```python
from build123d import *

# Parameters (mm, degrees)
SKETCH1_W           = 121
SKETCH1_H           = 25
BOSS_EXTRUDE1_DEPTH = 4
SKETCH3_W           = 10
SKETCH3_H           = 4
BOSS_EXTRUDE3_DEPTH = 4
LPATTERN2_COUNT     = 3
LPATTERN2_PITCH     = 20
LPATTERN2_COL_COUNT = 3
LPATTERN2_COL_PITCH = 20
SKETCH4_W           = 4
SKETCH4_H           = 5
BOSS_EXTRUDE4_DEPTH = 4
LPATTERN3_COUNT     = 3
LPATTERN3_PITCH     = 10


with BuildPart() as part:
    # Sketch1 → Boss-Extrude1 (new body)
    with BuildSketch(Plane(origin=(0, 0, 0), x_dir=(1, 0, 0), z_dir=(0, 1, 0))):
        with Locations((60.5, -12.5)):
            Rectangle(SKETCH1_W, SKETCH1_H)
    extrude(amount=BOSS_EXTRUDE1_DEPTH)

    # Sketch3 → Boss-Extrude3 (add, through all)
    with BuildSketch(Plane(origin=(0, 0, 0), x_dir=(-1, 0, 0), z_dir=(0, -1, 0))):
        with Locations((-60.5, 2)):
            Rectangle(SKETCH3_W, SKETCH3_H)
    boss_extrude3 = extrude(amount=-BOSS_EXTRUDE3_DEPTH)

    # LPattern2: Boss-Extrude3 ×3
    with Locations(*[(i * LPATTERN2_PITCH, 0, 0) for i in range(1, LPATTERN2_COUNT)]):
        add(boss_extrude3)

    # LPattern2 col: Boss-Extrude3 ×3
    with Locations(*[(-i * LPATTERN2_COL_PITCH, 0, 0) for i in range(1, LPATTERN2_COL_COUNT)]):
        add(boss_extrude3)

    # Sketch4 → Boss-Extrude4 (add, through all)
    with BuildSketch(Plane(origin=(0, 4, 0), x_dir=(1, 0, 0), z_dir=(0, 1, 0))):
        with Locations((-2, -22.5)):
            Rectangle(SKETCH4_W, SKETCH4_H)
        with Locations((123, -22.5)):
            Rectangle(SKETCH4_W, SKETCH4_H)
    boss_extrude4 = extrude(amount=-BOSS_EXTRUDE4_DEPTH)

    # LPattern3: Boss-Extrude4 ×3
    with Locations(*[(0, 0, -i * LPATTERN3_PITCH) for i in range(1, LPATTERN3_COUNT)]):
        add(boss_extrude4)


solid = part.part
```
The listing builds one solid part. Answer for the finished solid, in the listing's coordinates (mm). A direction names the side the tool comes from. Round coordinates to 2 decimals unless told otherwise and drop trailing zeros. Order: outer loops, then holes, each group sorted by start corner. A loop starts at its lowest first (then second) coordinate and runs counter-clockwise, first axis right, second up. Notation, with made-up numbers: (-12, 46.25) - (25, 46.25) arc R13 ccw to (25, 59.25) - close; hole circle Ø3 at (-1.75, 4). An arc over 180 degrees is marked (long way). Put each result on its own line as item: value. Start each with the question number.
(1) Find section A-A (x = 113). Give the vertices of the cut face in (y, z), plus the area to 3 significant figures.
(2) Determine the mould class of faces 4 (the flat face through (121, 2, 8)), 5 (the flat face through (-4, 2, 13)), 6 (the flat face through (81, 2, -4)) for opening direction Z: released by +Z, released by -Z, zero draft, split by the parting line, or undercut.
(3) Straight lines are drawn through the part: probe 1 along Z at (x, y) = (49.5, 1.6); probe 2 along X at (y, z) = (1.65, 9.75). For each, find the intervals that lie inside material, in ascending order. Write a range as from..to.
(4) For faces 1 (the flat face through (-2, 2, 10)), 2 (the flat face through (115, 2, 0)), 3 (the flat face through (90, 2, 0)), determine the directions among +Z, -Z, +X, -X, +Y, -Y from which every point of the face is accessible in a straight line to the end or side of a thin tool.
(5) Given P1, Ø2, axis at y = 2.5, z = 7.5, coming from the +X side; P2, Ø2, axis at x = -2, y = 3, coming from the -Z side; P3, Ø2, axis at y = 2, z = -1.5, coming from the -X side, each flat-ended and moving along its own axis, determine where each tip first touches the part or whether it passes through.
Reply:
1. outline: (0, 0) - (4, 0) - (4, 25) - (0, 25) - close
1. area: 100 mm^2
2. face 4: undercut
2. face 5: zero draft
2. face 6: released by -Z
3. probe 1: 0..25
3. probe 2: 0..121
4. face 1: -X, +Y, -Y
4. face 2: -Z, +X, +Y, -Y
4. face 3: -Z, +Y, -Y
5. P1: x = 121
5. P2: z = 0
5. P3: x = 15.5
